For this review, take the finished solid that the model builds, in its own axes (mm). Face numbers are marked on the shaded views. A direction names the side the tool comes from. Round coordinates to 2 decimals unless told otherwise and drop trailing zeros. Loops run counter-clockwise (first coordinate to the right, second up) from the corner with the lowest first, then second, coordinate; pieces in that order, holes last.
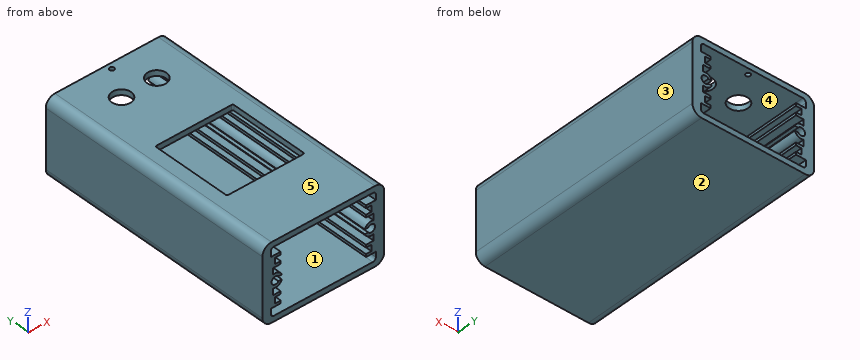
```python
from build123d import *

# Parameters (mm, degrees)
EXTRUDE_1_DEPTH     = 80
CUT_EXTRUDE_1_REACH = 88.168
CUT_EXTRUDE_2_REACH = 88.168
SKETCH_3_R          = 3.15
CUT_EXTRUDE_3_REACH = 88.168
SKETCH_4_R          = 0.75


with BuildPart() as part:
    # 草图1 → 凸台-拉伸1 (new body)
    with BuildSketch(Plane(origin=(0, 0, 0), x_dir=(1, 0, 0), z_dir=(0, 1, 0))):
        with BuildLine():
            Line((-17, 12.5), (17, 12.5))
            ThreePointArc((17, 12.5), (19.121320344, 11.621320344), (20, 9.5))
            Line((20, 9.5), (20, -9.5))
            ThreePointArc((20, -9.5), (19.121320344, -11.621320344), (17, -12.5))
            Line((17, -12.5), (-17, -12.5))
            ThreePointArc((-17, -12.5), (-19.121320344, -11.621320344), (-20, -9.5))
            Line((-20, -9.5), (-20, 9.5))
            ThreePointArc((-20, 9.5), (-19.121320344, 11.621320344), (-17, 12.5))
        make_face()
        with BuildLine():
            Line((-17.25, 8), (-14, 8))
            Line((-14, 8), (-14, 7.1))
            Line((-14, 7.1), (-15.8, 7.1))
            Line((-15.8, 7.1), (-15.8, 5.1))
            Line((-15.8, 5.1), (-14, 5.1))
            Line((-14, 5.1), (-14, 4.2))
            Line((-14, 4.2), (-16.5, 4.2))
            Line((-16.5, 4.2), (-16.5, 2.121320344))
            ThreePointArc((-16.5, 2.121320344), (-14.780330086, 2.030330086), (-13.628679656, 0.75))
            Line((-13.628679656, 0.75), (-14.75, 0.75))
            ThreePointArc((-14.75, 0.75), (-17, 0), (-14.75, -0.75))
            Line((-14.75, -0.75), (-13.628679656, -0.75))
            ThreePointArc((-13.628679656, -0.75), (-14.780330086, -2.030330086), (-16.5, -2.121320344))
            Line((-16.5, -2.121320344), (-16.5, -4.2))
            Line((-16.5, -4.2), (-14, -4.2))
            Line((-14, -4.2), (-14, -5.1))
            Line((-14, -5.1), (-15.8, -5.1))
            Line((-15.8, -5.1), (-15.8, -7.1))
            Line((-15.8, -7.1), (-14, -7.1))
            Line((-14, -7.1), (-14, -8))
            Line((-14, -8), (-17.25, -8))
            Line((-17.25, -8), (-17.25, -9.7))
            ThreePointArc((-17.25, -9.7), (-16.957106781, -10.407106781), (-16.25, -10.7))
            Line((-16.25, -10.7), (16.25, -10.7))
            ThreePointArc((16.25, -10.7), (16.957106781, -10.407106781), (17.25, -9.7))
            Line((17.25, -9.7), (17.25, -8))
            Line((17.25, -8), (14, -8))
            Line((14, -8), (14, -7.1))
            Line((14, -7.1), (15.8, -7.1))
            Line((15.8, -7.1), (15.8, -5.1))
            Line((15.8, -5.1), (14, -5.1))
            Line((14, -5.1), (14, -4.2))
            Line((14, -4.2), (16.5, -4.2))
            Line((16.5, -4.2), (16.5, -2.121320344))
            ThreePointArc((16.5, -2.121320344), (14.780330086, -2.030330086), (13.628679656, -0.75))
            Line((13.628679656, -0.75), (14.75, -0.75))
            ThreePointArc((14.75, -0.75), (17, 0), (14.75, 0.75))
            Line((14.75, 0.75), (13.628679656, 0.75))
            ThreePointArc((13.628679656, 0.75), (14.780330086, 2.030330086), (16.5, 2.121320344))
            Line((16.5, 2.121320344), (16.5, 4.2))
            Line((16.5, 4.2), (14, 4.2))
            Line((14, 4.2), (14, 5.1))
            Line((14, 5.1), (15.8, 5.1))
            Line((15.8, 5.1), (15.8, 7.1))
            Line((15.8, 7.1), (14, 7.1))
            Line((14, 7.1), (14, 8))
            Line((14, 8), (17.25, 8))
            Line((17.25, 8), (17.25, 9.7))
            ThreePointArc((17.25, 9.7), (16.957106781, 10.407106781), (16.25, 10.7))
            Line((16.25, 10.7), (-16.25, 10.7))
            ThreePointArc((-16.25, 10.7), (-16.957106781, 10.407106781), (-17.25, 9.7))
            Line((-17.25, 9.7), (-17.25, 8))
        make_face(mode=Mode.SUBTRACT)
    extrude(amount=EXTRUDE_1_DEPTH)

    # 草图2 → 切除-拉伸1 (cut, up to next)
    with BuildSketch(Plane.XY.offset(12.5), mode=Mode.PRIVATE) as cut_extrude_1_sk1:
        with BuildLine():
            Line((-12.25, 47.74), (12.25, 47.74))
            ThreePointArc((12.25, 47.74), (12.603553391, 47.593553391), (12.75, 47.24))
            Line((12.75, 47.24), (12.75, 21.74))
            ThreePointArc((12.75, 21.74), (12.603553391, 21.386446609), (12.25, 21.24))
            Line((12.25, 21.24), (-12.25, 21.24))
            ThreePointArc((-12.25, 21.24), (-12.603553391, 21.386446609), (-12.75, 21.74))
            Line((-12.75, 21.74), (-12.75, 47.24))
            ThreePointArc((-12.75, 47.24), (-12.603553391, 47.593553391), (-12.25, 47.74))
        make_face()
    cut_extrude_1_tool1 = extrude(cut_extrude_1_sk1.sketch, amount=-CUT_EXTRUDE_1_REACH, mode=Mode.PRIVATE) & part.part
    add(cut_extrude_1_tool1.solids().sort_by_distance((0, 34.49, 12.5))[0], mode=Mode.SUBTRACT)

    # 草图3 → 切除-拉伸2 (cut, up to next)
    with BuildSketch(Plane.XY.offset(12.5), mode=Mode.PRIVATE) as cut_extrude_2_sk1:
        with Locations((-5.8, 68)):
            Circle(SKETCH_3_R)
    cut_extrude_2_tool1 = extrude(cut_extrude_2_sk1.sketch, amount=-CUT_EXTRUDE_2_REACH, mode=Mode.PRIVATE) & part.part
    # 草图3 → 切除-拉伸2 (cut, up to next)
    with BuildSketch(Plane.XY.offset(12.5), mode=Mode.PRIVATE) as cut_extrude_2_sk2:
        with Locations((5.8, 68)):
            Circle(SKETCH_3_R)
    cut_extrude_2_tool2 = extrude(cut_extrude_2_sk2.sketch, amount=-CUT_EXTRUDE_2_REACH, mode=Mode.PRIVATE) & part.part
    add(cut_extrude_2_tool1.solids().sort_by_distance((-5.8, 68, 12.5))[0], mode=Mode.SUBTRACT)
    add(cut_extrude_2_tool2.solids().sort_by_distance((5.8, 68, 12.5))[0], mode=Mode.SUBTRACT)

    # 草图4 → 切除-拉伸3 (cut, up to next)
    with BuildSketch(Plane.XY.offset(12.5), mode=Mode.PRIVATE) as cut_extrude_3_sk1:
        with Locations((0, 78.1)):
            Circle(SKETCH_4_R)
    cut_extrude_3_tool1 = extrude(cut_extrude_3_sk1.sketch, amount=-CUT_EXTRUDE_3_REACH, mode=Mode.PRIVATE) & part.part
    add(cut_extrude_3_tool1.solids().sort_by_distance((0, 78.1, 12.5))[0], mode=Mode.SUBTRACT)


solid = part.part
```
(1) Add section C-C (z = -8.75). Give the boundary of the cut face in (x, y).
(2) Add section A-A (z = 0). Give the boundary of the cut face in (x, y), plus the area to 3 significant figures.
(3) For the marked faces 4 and 5, list the 3-axis set-ups (+Z, -Z, +X, -X, +Y, -Y) from which the entire face can be reached by the end or side of a thin tool; tool diameter is ignored.
(4) Add section D-D (x = 4). Give the boundary of the cut face in (y, z), plus the area to 3 significant figures.
(5) Add section B-B (x = -5.8). Give the boundary of the cut face in (y, z).
(6) Insertion check: pin 1 Ø2 at (x, y) = (11.5, 33.5) entering from +Z; pin 2 Ø10 at (x, z) = (-10.5, 6.5) entering from +Y; pin 3 Ø2 at (y, z) = (39, 12) entering from -X. Each pin has a flat end and moves straight along its axis. Give the tip position at first contact, or say it passes through.
(7) The part is to be moulded in two halves that separate along X. For the marked faces 1, 2 and 3, say which applies: pulls with the +X half, pulls with the -X half, needs draft (parallel to the pull), parting line crosses it, or undercut.
(8) For L1, parallel to Y at x = 0, z = 12.1; L2, parallel to X at y = 36.5, z = 3.75; L3, parallel to Z at x = 0.5, y = 72.5, list the stretches that pass through material, from the lowest coordinate up.
Outcome:
1. outline: (-20, 0) - (-17.25, 0) - (-17.25, 80) - (-20, 80) - close; (17.25, 0) - (20, 0) - (20, 80) - (17.25, 80) - close
2. outline: (-20, 0) - (-17, 0) - (-17, 80) - (-20, 80) - close; (17, 0) - (20, 0) - (20, 80) - (17, 80) - close
2. area: 480 mm2
3. face 4: +Y, -Y
3. face 5: +Z, +X, -X, +Y, -Y
4. outline: (0, -12.5) - (80, -12.5) - (80, -10.7) - (0, -10.7) - close; (0, 10.7) - (21.24, 10.7) - (21.24, 12.5) - (0, 12.5) - close; (47.74, 10.7) - (65.41, 10.7) - (65.41, 12.5) - (47.74, 12.5) - close; (70.59, 10.7) - (80, 10.7) - (80, 12.5) - (70.59, 12.5) - close
4. area: 231 mm2
5. outline: (0, -12.5) - (80, -12.5) - (80, -10.7) - (0, -10.7) - close; (0, 10.7) - (21.24, 10.7) - (21.24, 12.5) - (0, 12.5) - close; (47.74, 10.7) - (64.85, 10.7) - (64.85, 12.5) - (47.74, 12.5) - close; (71.15, 10.7) - (80, 10.7) - (80, 12.5) - (71.15, 12.5) - close
6. pin 1: stops at z = -10.7
6. pin 2: stops at y = 80
6. pin 3: stops at x = -19.6
7. face 1: undercut
7. face 2: needs draft
7. face 3: pulls with the +X half
8. L1: y = 0 to 21.24, 47.74 to 77.35, 78.85 to 80
8. L2: x = -20 to -16.5, 16.5 to 20
8. L3: z = -12.5 to -10.7, 10.7 to 12.5
